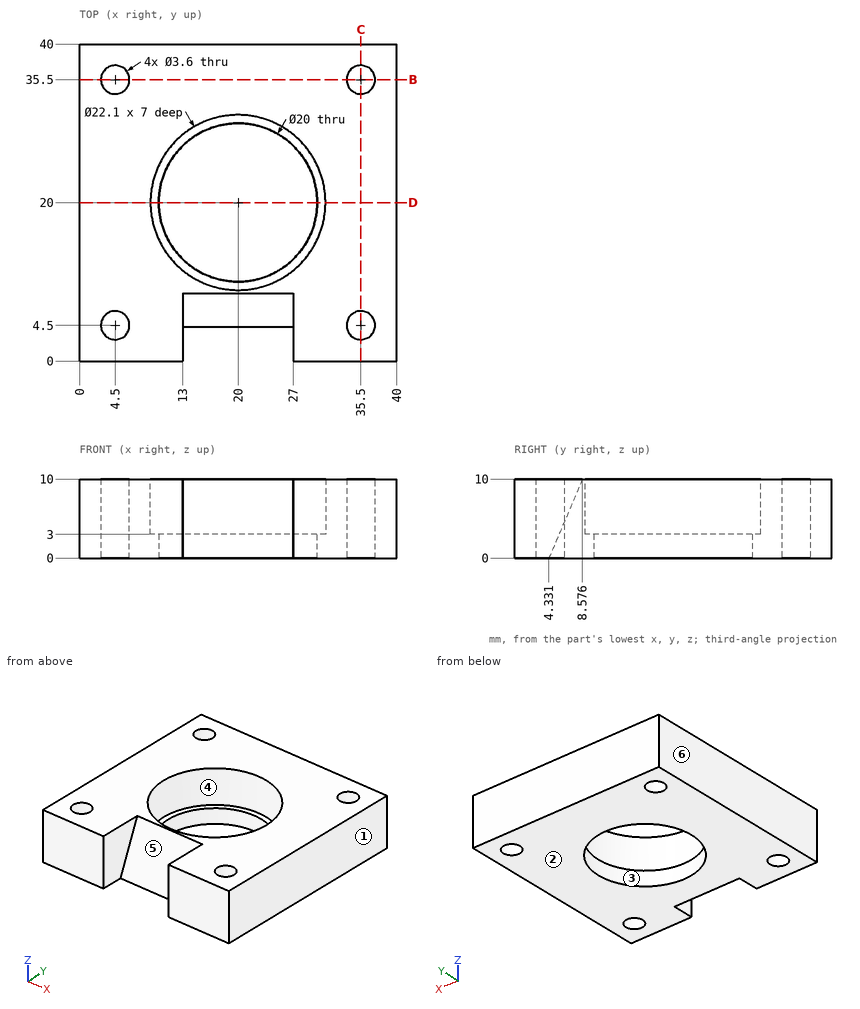
Input: dimensioned drawing with shaded views. Units: mm. Origin: part minimum x, y, z. A direction names the side the tool comes from. Give positions to 0.01 mm unless a question says otherwise; leave off trailing zeros. Write each loop counter-clockwise with the first axis right and the second up, starting at its lowest first coordinate (ties: lowest second). Pieces come first, ordered by that corner, then holes. Notation, with made-up numbers: (30, 83) -> (36, 83) arc R23 cw to (36, 112) -> close; hole circle Ø10 at (10, 41). An arc over 180 degrees is marked (long way). Answer as a JSON object with one key per item and string values.
1. Cut plane B-B on y = 35.5. Output: boundary loops of the cut face in (x, z).
Ans:
{"outline": "(0, 0) -> (2.7, 0) -> (2.7, 10) -> (0, 10) -> close; (6.3, 0) -> (33.7, 0) -> (33.7, 10) -> (6.3, 10) -> close; (37.3, 0) -> (40, 0) -> (40, 10) -> (37.3, 10) -> close"}
2. Ray query, probe 1 along Y at (x, z) = (35.5, 8.25); probe 2 along Y at (x, z) = (34.5, 8.5) (1 decimal); probe 3 along X at (y, z) = (5, 8.25). Return the intervals inside material, ascending. Write a range as from..to.
Ans:
{"probe 1": "y = 0..2.7, 6.3..33.7, 37.3..40", "probe 2": "y = 0..3, 6..34, 37..40", "probe 3": "x = 0..2.77, 6.23..13, 27..33.77, 37.23..40"}
3. Access query for the marked faces 4, 5 and 6. Directions: +Z, -Z, +X, -X, +Y, -Y. A direction counts if a zero-diameter tool reaches every point of the face in a straight line with its end or side. Return the directions, or none.
Ans:
{"face 4": "+Z", "face 5": "+Z, -Y", "face 6": "+Z, -Z, -X, +Y, -Y"}
4. Mould query, pull axis X, two halves, no side actions, for the marked faces 1, 2 and 3. Classes: pulls with the +X half, pulls with the -X half, needs draft (parallel to the pull), parting line crosses it, or undercut.
Ans:
{"face 1": "pulls with the +X half", "face 2": "needs draft", "face 3": "undercut"}
5. Cut plane D-D on y = 20. Output: boundary loops of the cut face in (x, z).
Ans:
{"outline": "(0, 0) -> (10, 0) -> (10, 3) -> (8.95, 3) -> (8.95, 10) -> (0, 10) -> close; (30, 0) -> (40, 0) -> (40, 10) -> (31.05, 10) -> (31.05, 3) -> (30, 3) -> close"}
6. Contact query for flat-ended pins moving along their axis: pin 1 (2 mm diameter, centred on x = 35.5, y = 35.5, fed in from -Z); pin 2 (5 mm diameter, centred on x = 16, z = 6, fed in from -Y). Output: stop coordinate, or through.
Ans:
{"pin 1": "passes through", "pin 2": "stops at y = 5.82"}
